Could you check a few things on this drawing? It's one solid part, dimensions in mm from its lowest x, y, z. Give positions to 0.01 mm unless a question says otherwise; leave off trailing zeros. Loops run counter-clockwise (first coordinate to the right, second up) from the corner with the lowest first, then second, coordinate; pieces in that order, holes last. Notation, with made-up numbers: M 14,11 L 60,11 A36 cw 60,48 Z; hole C 84,-32.75 d7. An arc over 180 degrees is marked long. Answer as a JSON object with one key per item and string values.
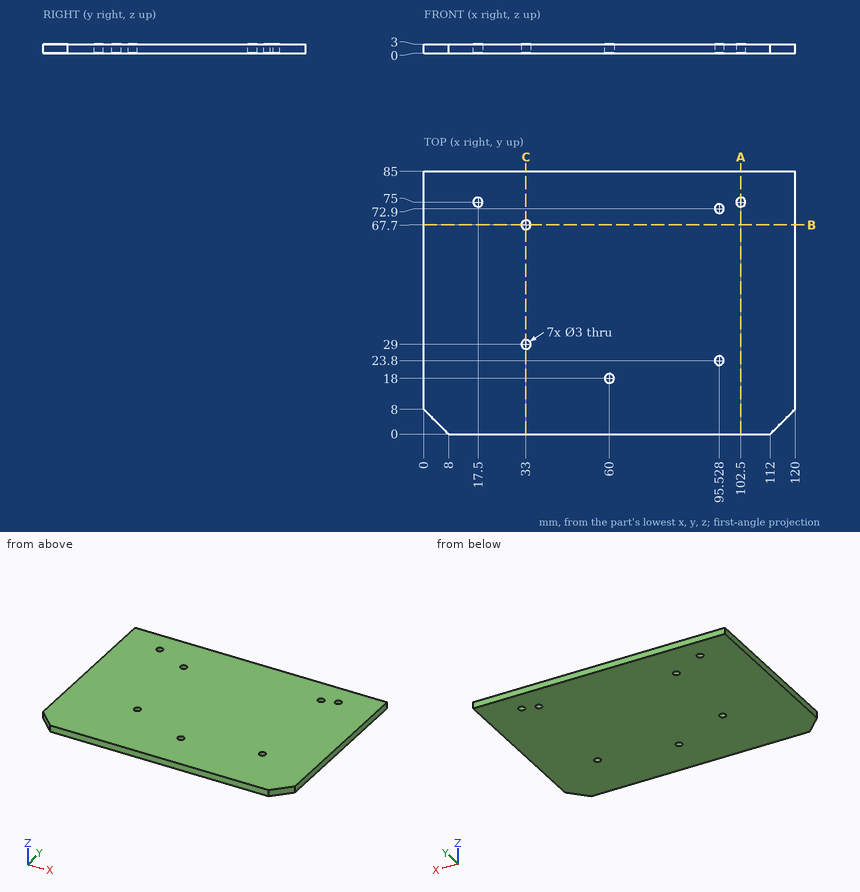
1) Suppose I cut it at A-A, the plane x = 102.5. Write out the boundary of the cut face in (y, z), and give its area (3 significant figures).
Answer list:
{"outline": "M 0,0 L 73.5,0 L 73.5,3 L 0,3 Z; M 76.5,0 L 85,0 L 85,3 L 76.5,3 Z", "area": "246 mm^2"}
2) Suppose I cut it at B-B, the plane y = 67.7. Write out the boundary of the cut face in (x, z).
Answer list:
{"outline": "M 0,0 L 31.5,0 L 31.5,3 L 0,3 Z; M 34.5,0 L 120,0 L 120,3 L 34.5,3 Z"}
3) Please list where these lines run through material, in increasing order: line 1 along Y through (x, z) = (33, 2); line 2 along X through (y, z) = (29, 2); line 3 along X through (y, z) = (75, 2.2). Write a range as from..to.
Answer list:
{"line 1": "0..27.5, 30.5..66.2, 69.2..85", "line 2": "0..31.5, 34.5..120", "line 3": "0..16, 19..101, 104..120"}
4) Suppose I cut it at C-C, the plane x = 33. Write out the boundary of the cut face in (y, z), and give its area (3 significant figures).
Answer list:
{"outline": "M 0,0 L 27.5,0 L 27.5,3 L 0,3 Z; M 30.5,0 L 66.2,0 L 66.2,3 L 30.5,3 Z; M 69.2,0 L 85,0 L 85,3 L 69.2,3 Z", "area": "237 mm^2"}
5) Will this pin go through, and if not, where does the flat tip stop? pin 1 Ø2.5 at (x, y) = (17.5, 75) entering from +Z.
Answer list:
{"pin 1": "through"}
